Geometry check sheet. Reference: the model listing, model coordinates, mm. Round coordinates to 2 decimals unless told otherwise and drop trailing zeros. Order: outer loops, then holes, each group sorted by start corner. A loop starts at its lowest first (then second) coordinate and runs counter-clockwise, first axis right, second up. Notation, with made-up numbers: (53, 35.5) -> (62, 35.5) arc R20 cw to (62, 72.5) -> close; hole circle Ø8 at (34.25, 59.5). An arc over 180 degrees is marked (long way). Answer as a JSON object with one key per item and string values. Group by question number.
from build123d import *

# Parameters (mm, degrees)
SKETCH1_R           = 11.176
BOSS_EXTRUDE1_DEPTH = 513.588
SKETCH2_W           = 511.048
SKETCH2_H           = 1.5875
CUT_EXTRUDE1_DEPTH  = 5.08


with BuildPart() as part:
    # Sketch1 → Boss-Extrude1 (new body)
    with BuildSketch(Plane.XY):
        with BuildLine():
            Line((0, -12.7), (-12.7, -12.7))
            Line((-12.7, -12.7), (-12.7, -10.0965))
            Line((-12.7, -10.0965), (-7.703939755, -10.0965))
            ThreePointArc((-7.703939755, -10.0965), (4.065983891, 12.031532529), (0, -12.7))
        make_face()
        Circle(SKETCH1_R, mode=Mode.SUBTRACT)
    extrude(amount=BOSS_EXTRUDE1_DEPTH)

    # Sketch2 → Cut-Extrude1 (cut)
    with BuildSketch(Plane.ZY.offset(12.7)):
        with Locations((256.794, -11.39825)):
            Rectangle(SKETCH2_W, SKETCH2_H)
    extrude(amount=-CUT_EXTRUDE1_DEPTH, mode=Mode.SUBTRACT)


solid = part.part
Item 1: Sectioned sample at C-C, the plane x = 5.5. Enter the section's corners in (y, z).
Item 2: Sectioned sample at B-B, the plane z = 411.5. Enter the section's corners in (x, y), then the cut area to 3 significant figures.
Item 3: Mould release check, pull along X, two halves, no side actions. Record for faces 1 (the cylindrical face through (-8.87, -6.8, 253.2)), 2 (the flat face through (-6, -10, 513.588)): pulls with the +X half, pulls with the -X half, needs draft (parallel to the pull), parting line crosses it, or undercut.
Item 4: Depth check by flat-ended pin: pin 1 Ø4 at (x, z) = (-11, 351) entering from +Y; pin 2 Ø5 at (x, y) = (-1.5, 6) entering from +Z; pin 3 Ø2 at (x, z) = (6.5, 137.5) entering from -Y; pin 4 Ø1 at (x, z) = (-2, 81.5) entering from +Y. Enter the tip coordinate at first touch or a pass-through.
Item 5: Sectioned sample at A-A, the plane y = 0. Enter the section's corners in (x, z).
Item 6: Thickness scan on L1, parallel to Y at x = 1.5, z = 151; L2, parallel to X at y = 0.5, z = 333; L3, parallel to X at y = -0.75, z = 441. Record the ranges inside material, lowest first.
Result:
{
 "1": {"outline": "(-11.45, 0) -> (-9.73, 0) -> (-9.73, 513.59) -> (-11.45, 513.59) -> close; (9.73, 0) -> (11.45, 0) -> (11.45, 513.59) -> (9.73, 513.59) -> close"},
 "2": {"outline": "(-12.7, -12.7) -> (0, -12.7) arc R12.7 ccw (long way) to (-7.7, -10.1) -> (-12.7, -10.1) -> (-12.7, -10.6) -> (-7.62, -10.6) -> (-7.62, -12.19) -> (-12.7, -12.19) -> close; hole circle Ø22.35 at (0, 0)", "area": "126 mm2"},
 "3": {"face 1": "undercut", "face 2": "needs draft"},
 "4": {"pin 1": "stops at y = 8.96", "pin 2": "passes through", "pin 3": "stops at y = -11.45", "pin 4": "stops at y = 12.61"},
 "5": {"outline": "(-12.7, 0) -> (-11.18, 0) -> (-11.18, 513.59) -> (-12.7, 513.59) -> close; (11.18, 0) -> (12.7, 0) -> (12.7, 513.59) -> (11.18, 513.59) -> close"},
 "6": {"L1": "y = -12.61 to -11.07, 11.07 to 12.61", "L2": "x = -12.69 to -11.16, 11.16 to 12.69", "L3": "x = -12.68 to -11.15, 11.15 to 12.68"}
}
